Design review of the part built by this model. Coordinates are the model's own, in mm. A direction names the side the tool comes from. Round coordinates to 2 decimals unless told otherwise and drop trailing zeros. Order: outer loops, then holes, each group sorted by start corner. A loop starts at its lowest first (then second) coordinate and runs counter-clockwise, first axis right, second up. Notation, with made-up numbers: M 48,45.25 L 93,45.25 A19 ccw 93,73.25 Z; hole C -27,75.25 d10. An arc over 180 degrees is marked long. Write each question's results on one line, items separated by ' | '. Start each with the question number.
Item 1: Clearance check with flat-ended pins moving along their axes: pin 1 (1.9 mm diameter, centred on x = 1.5, z = 0.5, fed in from +Y); pin 2 (2 mm diameter, centred on x = -0.5, y = 21.5, fed in from -Z); pin 3 (4 mm diameter, centred on y = 32.5, z = 1, fed in from +X). State where each tip first meets the part, or that it passes through.
Item 2: The part is to be moulded in two halves that separate along X. For faces 1 (the cylindrical face through (0.69, 30.42, 3.1)), 2 (the cylindrical face through (0.77, 52.696, -5.868)), 3 (the flat face through (3, 53.34, 3)), say which applies: +X half, -X half, draft (parallel to the pull), parting line (faces both ways), or undercut.
Item 3: Machinability: for faces 4 (the flat face through (0, 6.858, 0)), 5 (the flat face through (0, 0, 0)), 6 (the cylindrical face through (1.008, 24.014, 4.538)), which of the approach directions +Z, -Z, +X, -X, +Y, -Y give a long, thin tool a straight path to every point of the face, cutting with its end or side? Answer none if there is none.
Item 4: Take a section at B-B, the plane x = 0. Write out the cut boundary in (y, z) (3 decimals).
Item 5: Take a section at C-C, the plane y = 45.5. Write out the cut boundary in (x, z) (3 decimals).
Item 6: Take a section at A-A, the plane z = 0. Write out the cut boundary in (x, y) (3 decimals), plus the area to 3 significant figures.
Item 7: Wall thickness on line 1 (Z direction, x = 0, y = 24) (3 decimals); line 2 (Y direction, x = -2.5, z = 0): over which ranges is each line inside the solid? List them lowest first. Write a range as [from, to].
```python
from build123d import *


# Not quite as in the source:
# - a fillet or chamfer that OpenCascade refuses, or shapes differently, is made with other operations: its cross-section is extruded or revolved along the edge and cut away or added


with BuildPart() as f1:
    # F0 (on Top) → F1 (revolve)
    with BuildSketch(Plane.XY):
        Polygon((-4.6482, 0), (0, 0), (0, 6.8579994701), (-3.175, 6.8579994701), (-3.175, 53.34), (-4.6482, 53.34), (-5.9182, 53.34), (-5.9182, 52.07), (-4.6482, 52.07), align=None)
    revolve(axis=Axis((0, 3.4289997351, 0), (0, -1, 0)))

    # F2: fillet of radius 5.08 on 1 edges, made by hand

    # F2_s1 → F2_t2 (revolve)
    with BuildSketch(Plane.XY):
        with BuildLine():
            ThreePointArc((-5.9182, 52.07), (-4.9762951188, 50.5059470592), (-4.6482, 48.7098958349))
            Line((-4.6482, 48.7098958349), (-4.6482, 52.07))
            Line((-4.6482, 52.07), (-5.9182, 52.07))
        make_face()
    revolve(axis=Axis((0, 52.07, 0), (0, -1, 0)))


solid = f1.part
```
Results list:
1) pin 1: y = 6.86 | pin 2: z = -4.65 | pin 3: x = 4.65
2) face 1: undercut | face 2: parting line | face 3: draft
3) face 4: +Y | face 5: +Z, -Z, +X, -X, -Y | face 6: -Y
4) outline: M 0,-4.648 L 48.71,-4.648 A5.08 cw 52.07,-5.918 L 53.34,-5.918 L 53.34,-3.175 L 6.858,-3.175 L 6.858,3.175 L 53.34,3.175 L 53.34,5.918 L 52.07,5.918 A5.08 cw 48.71,4.648 L 0,4.648 Z
5) outline: C 0,0 d9.296; hole C 0,0 d6.35
6) outline: M -5.918,52.07 A5.08 cw -4.648,48.71 L -4.648,0 L 4.648,0 L 4.648,48.71 A5.08 cw 5.918,52.07 L 5.918,53.34 L 3.175,53.34 L 3.175,6.858 L -3.175,6.858 L -3.175,53.34 L -5.918,53.34 Z | area: 207 mm²
7) line 1: [-4.648, -3.175], [3.175, 4.648] | line 2: [0, 6.86]
